from build123d import *

# Parameters (mm, degrees)
ESBO_O1_W                = 5
ESBO_O1_H                = 4.35
RESSALTO_EXTRUS_O1_DEPTH = 120
RESSALTO_EXTRUS_O2_DEPTH = 4.35
CUT_EXTRUDE2_DEPTH       = 10
CUT_EXTRUDE3_DEPTH       = 10
SKETCH17_W               = 1.7804771699968711
SKETCH17_H               = 4.499999999999998
BOSS_EXTRUDE2_DEPTH      = 1.5
FILLET8_R                = 1
FILLET9_R                = 0.5


with BuildPart() as part:
    # Esboço1 → Ressalto-extrusão1 (new body)
    with BuildSketch(Plane(origin=(0, 0, 0), x_dir=(0, 0, -1), z_dir=(1, 0, 0))):
        with Locations((-2.5000000000000098, 0)):
            Rectangle(ESBO_O1_W, ESBO_O1_H)
    extrude(amount=RESSALTO_EXTRUS_O1_DEPTH)

    # Esboço2 → Ressalto-extrusão2 (add)
    with BuildSketch(Plane(origin=(0, 2.175, 0), x_dir=(1, 0, 0), z_dir=(0, 1, 0))):
        Polygon((75, -9.63e-15), (87.5, -9.63e-15), (86.75, 4.49999999999999), align=None)
    extrude(amount=-RESSALTO_EXTRUS_O2_DEPTH)

    # Sketch12 → Cut-Extrude2 (cut)
    with BuildSketch(Plane(origin=(0, 2.175, 0), x_dir=(1, 0, 0), z_dir=(0, 1, 1.7e-16))):
        with BuildLine():
            Line((120, -2.5000000000000098), (108.78052366211932, -2.500000000000011))
            ThreePointArc((108.78052366211932, -2.500000000000011), (105.97177980074898, -1.8405473191538975), (103.75, -2.99e-15))
            Line((103.75, -2.99e-15), (120, -9.22e-15))
            Line((120, -9.22e-15), (120, -2.5000000000000098))
        make_face()
    extrude(amount=-CUT_EXTRUDE2_DEPTH, mode=Mode.SUBTRACT)

    # Fillet5
    # a fillet whose section is not a circle: 2 mm, written as the material it takes off along each edge
    with BuildSketch(Plane(origin=(86.75, 8.293980956389628, -4.49999999999999), x_dir=(-0.9338567516961642, 0, 0.35764726660704255), z_dir=(0, -1, 0))) as fillet5_piece_1:
        with BuildLine():
            Bezier((2.4475923825558348, 0), (6.4e-16, -1.66e-15), (0.48769743446495956, -2.3985119727784827), weights=[1, 1.2654991217782485, 1])
            Line((0.48769743446495956, -2.3985119727784827), (0, 0))
            Line((0, 0), (2.4475923825558348, 0))
        make_face()
    extrude(amount=16.587961912779257, mode=Mode.SUBTRACT)

    # Fillet6
    # a fillet whose section is not a circle: 2 mm, written as the material it adds along each edge
    with BuildSketch(Plane(origin=(75, 2.175, 9.63e-15), x_dir=(-1, 0, -2e-17), z_dir=(0, -1, 0))) as fillet6_piece_1:
        with BuildLine():
            Bezier((0.36987979207182775, 0), (0, 1e-17), (-0.3454147411422639, 0.13228649660767453), weights=[1, 1.966650325653325, 1])
            Line((-0.3454147411422639, 0.13228649660767453), (0, 0))
            Line((0, 0), (0.36987979207182775, 0))
        make_face()
    extrude(amount=4.35)

    # Fillet7
    # a fillet whose section is not a circle: 2 mm, written as the material it adds along each edge
    with BuildSketch(Plane(origin=(87.5, 2.175, 9.63e-15), x_dir=(1, 0, -1e-17), z_dir=(0, -1, 0))) as fillet7_piece_1:
        with BuildLine():
            Bezier((1.69425417676608, 0), (0, -1e-17), (-0.2785336708982129, -1.671202025389285), weights=[1, 1.5260399649454515, 1])
            Line((-0.2785336708982129, -1.671202025389285), (0, 0))
            Line((0, 0), (1.69425417676608, 0))
        make_face()
    extrude(amount=4.35)

    # Sketch16 → Cut-Extrude3 (cut)
    with BuildSketch(Plane.XY):
        Polygon((23.000000000000007, -1.4999999999999984), (20.000000000000007, -1.499999999999998), (20.000000000000004, 1.500000000000001), (23.000000000000007, 1.5000000000000013), align=None)
        Polygon((18.000000000000004, -1.4999999999999978), (15.000000000000002, -1.4999999999999984), (14.999999999999998, 1.5000000000000007), (18.000000000000004, 1.5000000000000013), align=None)
        Polygon((13.000000000000004, -1.4999999999999958), (10.000000000000002, -1.4999999999999964), (10.000000000000005, 1.5000000000000029), (13.000000000000007, 1.5000000000000036), align=None)
        Polygon((8, -1.4999999999999956), (5.000000000000001, -1.4999999999999953), (4.999999999999997, 1.500000000000004), (7.9999999999999964, 1.5000000000000038), align=None)
    extrude(amount=CUT_EXTRUDE3_DEPTH, mode=Mode.SUBTRACT)

    # Sketch17 → Boss-Extrude2 (add)
    with BuildSketch(Plane(origin=(2.9e-16, -4.3e-16, 2.500000000000023), x_dir=(-1, 0, 0), z_dir=(0, 1.7e-16, -1))):
        with Locations((-119.10976141500157, -0.07499999999999951)):
            Rectangle(SKETCH17_W, SKETCH17_H)
    extrude(amount=BOSS_EXTRUDE2_DEPTH)

    # Fillet8
    fillet8_edges = [part.edges().sort_by_distance(p)[0] for p in [
        (118.21952283000314, -4.3e-16, 2.500000000000023),
    ]]
    fillet(fillet8_edges, radius=FILLET8_R)

    # Fillet9
    fillet9_edges = [part.edges().sort_by_distance(p)[0] for p in [
        (120, -0.07499999999999947, 1.000000000000023),
        (118.21952283000314, -0.07499999999999991, 1.000000000000023),
    ]]
    fillet(fillet9_edges, radius=FILLET9_R)


solid = part.part
Geometry check sheet. Reference: the model listing, model coordinates, mm. A direction names the side the tool comes from. Coordinates: 2 decimals unless noted, no trailing zeros. Order: outer loops, then holes, each group sorted by start corner. A loop starts at its lowest first (then second) coordinate and runs counter-clockwise, first axis right, second up. Notation, with made-up numbers: (-38, 70) - (10, 70) arc R26 cw to (10, 89) - close; hole circle Ø6 at (16.25, 33.5). An arc over 180 degrees is marked (long way). One line per item, written item: value.
(1) Thickness scan on probe 1 along X at (y, z) = (-0.65, 3.5); probe 2 along Y at (x, z) = (7, 2.25) (3 decimals); probe 3 along Y at (x, z) = (30.5, 1.5) (3 decimals). Record the ranges inside material, lowest first. Write a range as from..to.
Data:
probe 1: x = 0..5, 8..10, 13..15, 18..20, 23..120
probe 2: y = -2.175..-1.5, 1.5..2.175
probe 3: y = -2.175..2.175
(2) Sectioned sample at A-A (y = 0.2). Count the separate pieces of the cut face and the enclosed holes in it, and give its area (3 significant figures).
Data:
separate pieces: 5
enclosed holes: 0
area: 534 mm^2
(3) Depth check by flat-ended pin: pin 1 Ø1 at (x, z) = (34.5, 2) entering from -Y (3 decimals); pin 2 Ø2.5 at (y, z) = (0.5, 2.5) entering from -X. Enter the tip coordinate at first touch or a pass-through.
Data:
pin 1: stops at y = -2.175
pin 2: stops at x = 0
(4) Access from +Z, -Z, +X, -X, +Y, -Y to the whole of each face (thin tool, end or side, straight path). Record for faces 5 (the face through (106.01, 0.03, 1.86)), 6 (the face through (45, 0, 0)), 7 (the face through (20, 0, 2)).
Data:
face 5: -Z, +Y, -Y
face 6: -Z, -X, +Y, -Y
face 7: +Z, -Z
(5) Sectioned sample at B-B (x = 42.5). Enter the section's corners in (y, z) (3 decimals), and give its area (4 significant figures).
Data:
outline: (-2.175, 0) - (2.175, 0) - (2.175, 5) - (-2.175, 5) - close
area: 21.75 mm^2
(6) Release check for a two-part mould opening along X. For faces 1 (the face through (17, -1.5, 2)), 2 (the face through (11, 1.5, 2)), 3 (the face through (96, 0, 0)), 4 (the face through (0, 0, 3)) record: +X half, -X half, draft (parallel to the pull), parting line (faces both ways), or undercut.
Data:
face 1: undercut
face 2: undercut
face 3: draft
face 4: -X half
(7) Sectioned sample at C-C (x = 106.5). Enter the section's corners in (y, z) (3 decimals).
Data:
outline: (-2.175, 2.074) - (2.175, 2.074) - (2.175, 5) - (-2.175, 5) - close
